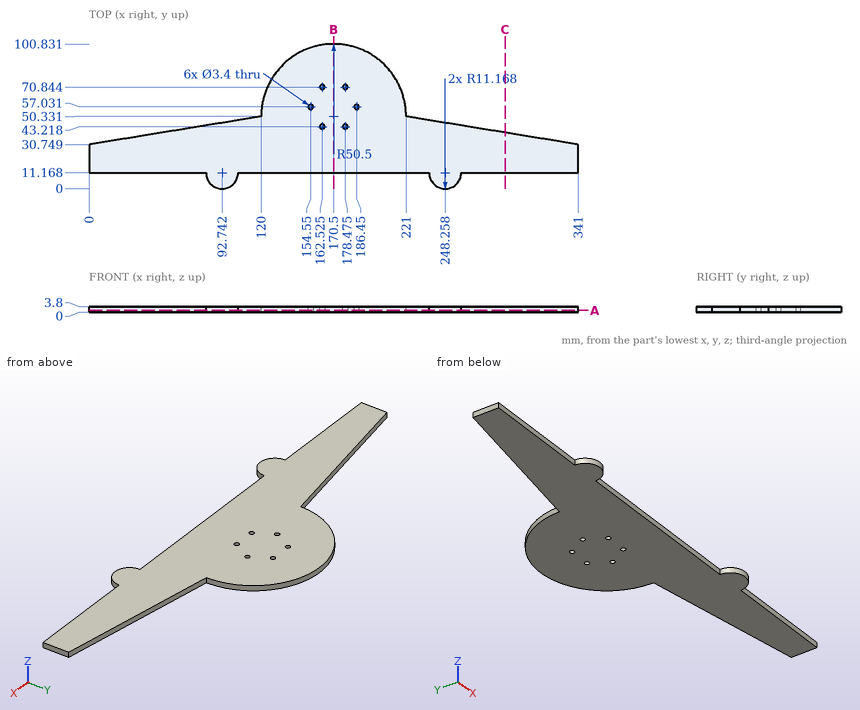
Geometry: see drawing. Coordinates: mm, zero at the bounding-box minimum. Coordinates: 2 decimals unless noted, no trailing zeros. Loops run counter-clockwise (first coordinate to the right, second up) from the corner with the lowest first, then second, coordinate; pieces in that order, holes last. Notation, with made-up numbers: (82.5, 20.25) - (113.5, 20.25) arc R16 ccw to (113.5, 31.25) - close; hole circle Ø11 at (79, 34). An arc over 180 degrees is marked (long way). Put each result on its own line as item: value. Start each with the question number.
Q1. Cut plane C-C, the plane x = 290. Return loops of the section in (y, z).
Q2. Line query: line 1 (X direction, y = 57, z = 0.5); line 2 (Y direction, x = 154.55, z = 1.35) (1 decimal); line 3 (Y direction, x = 165, z = 2.9). Output: solid intervals per line, ascending.
Q3. Cut plane B-B, the plane x = 170.5. Return loops of the section in (y, z).
Q4. Cut plane A-A, the plane z = 1.25. Give the number of separate pieces and of enclosed holes in the cut face, and give its area (3 significant figures).
Q5. Pin query (flat end, axial travel): pin 1 Ø2 at (y, z) = (58.5, 2) entering from +X; pin 2 Ø1.9 at (x, z) = (169.5, 2) entering from -Y. Return the tip coordinate at first contact, or that it passes through.
Filled sheet:
1. outline: (11.17, 0) - (39.07, 0) - (39.07, 3.8) - (11.17, 3.8) - close
2. line 1: 120.44 to 152.85, 156.25 to 184.75, 188.15 to 220.56
2. line 2: 11.2 to 55.3, 58.7 to 98.2
2. line 3: 11.17 to 100.53
3. outline: (11.17, 0) - (100.83, 0) - (100.83, 3.8) - (11.17, 3.8) - close
4. separate pieces: 1
4. enclosed holes: 6
4. area: 15,300 mm²
5. pin 1: x = 220.49
5. pin 2: y = 11.17
